from build123d import *

# Parameters (mm, degrees)
F0_R     = 34
F1_DEPTH = 5
F2_R     = 34
F2_R_2   = 3.2
F3_DEPTH = 5
F5_DEPTH = 10.001
F6_DEPTH = 4


with BuildPart() as f1:
    # F0 (on Top) → F1 (new body)
    with BuildSketch(Plane.XY):
        Circle(F0_R)
        Polygon((0, 5.34048999), (4.625, 2.670244995), (4.625, -2.670244995), (0, -5.34048999), (-4.625, -2.670244995), (-4.625, 2.670244995), align=None, mode=Mode.SUBTRACT)
    extrude(amount=F1_DEPTH)

    # F2 (on face) → F3 (join)
    with BuildSketch(Plane.XY.offset(5)):
        Circle(F2_R)
        Polygon((-4.625, -2.670244995), (-4.625, 2.670244995), (0, 5.34048999), (4.625, 2.670244995), (4.625, -2.670244995), (0, -5.34048999), align=None, mode=Mode.SUBTRACT)
        Polygon((0, 5.34048999), (-4.625, 2.670244995), (-4.625, -2.670244995), (0, -5.34048999), (4.625, -2.670244995), (4.625, 2.670244995), align=None)
        Circle(F2_R_2, mode=Mode.SUBTRACT)
    extrude(amount=F3_DEPTH)

    # F4 (on face) → F5 (cut, through all)
    with BuildSketch(Plane.XY.offset(10)):
        with BuildLine():
            ThreePointArc((34, 0), (25.9934550819, 21.9166670118), (5.7446886526, 33.5111705597))
            Line((5.7446886526, 33.5111705597), (31.8938693416, -11.7805389699))
            ThreePointArc((31.8938693416, -11.7805389699), (33.4693259389, -5.9836628575), (34, 0))
        make_face()
        with BuildLine():
            Line((-5.7446886526, -33.5111705597), (-31.8938693416, 11.7805389699))
            ThreePointArc((-31.8938693416, 11.7805389699), (-29.4448637287, -17), (-5.7446886526, -33.5111705597))
        make_face()
    extrude(amount=-F5_DEPTH, mode=Mode.SUBTRACT)

    # F4 (on face) → F6 (join)
    with BuildSketch(Plane.XY.offset(10)):
        with BuildLine():
            ThreePointArc((3.5, 33.8193731462), (1.7523288833, 33.9548132595), (0, 34))
            Line((0, 34), (0, 29.5))
            Line((0, 29.5), (3.5, 29.5))
            Line((3.5, 29.5), (3.5, 33.8193731462))
        make_face()
        with BuildLine():
            Line((-3.5, -29.5), (-3.5, -33.8193731462))
            ThreePointArc((-3.5, -33.8193731462), (-1.7523288833, -33.9548132595), (0, -34))
            Line((0, -34), (0, -29.5))
            Line((0, -29.5), (-3.5, -29.5))
        make_face()
    extrude(amount=F6_DEPTH)


solid = f1.part
Design review of the part built by this model. Coordinates are the model's own, in mm. A direction names the side the tool comes from. Coordinates: 2 decimals unless noted, no trailing zeros. Order: outer loops, then holes, each group sorted by start corner. A loop starts at its lowest first (then second) coordinate and runs counter-clockwise, first axis right, second up. Notation, with made-up numbers: M -20,13.5 L 19,13.5 A9 ccw 19,25.5 Z; hole C 68.25,36.5 d3. An arc over 180 degrees is marked long. Use a Markdown table: item, result.
(1) For P1, Ø2, axis at x = 13, y = 0, coming from the -Z side; P2, Ø2.5, axis at y = 0, z = 2, coming from the +X side; P3, Ø1, axis at x = -5.5, y = 15.5, coming from the +Z side; P4, Ø3, axis at x = 2, z = 12.5, coming from the -Y side, all flat-tipped, find the tip position at first contact; note any pin that passes through.
Worked answers:
| item | result |
|---|---|
| P1 | stops at z = 0 |
| P2 | stops at x = 25.81 |
| P3 | stops at z = 10 |
| P4 | stops at y = 29.5 |
(2) Add section A-A (z = 8.5). Give the boundary of the cut face in (x, y).
Worked answers:
| item | result |
|---|---|
| outline | M -31.89,11.78 L -5.74,-33.51 A34 ccw 31.89,-11.78 L 5.74,33.51 A34 ccw Z; hole C 0,0 d6.4 |
(3) Add section C-C (x = 7). Give the boundary of the cut face in (y, z).
Worked answers:
| item | result |
|---|---|
| outline | M -33.27,0 L 31.34,0 L 31.34,10 L -33.27,10 Z |
(4) Wall thickness on probe 1 along Y at (x, z) = (0, 6.25); probe 2 along Z at (x, y) = (-17, 5.5); probe 3 along Y at (x, z) = (3, 1.25): over which ranges is each line inside the solid? List them lowest first.
Worked answers:
| item | result |
|---|---|
| probe 1 | y = -34 to -3.2, 3.2 to 34 |
| probe 2 | z = 0 to 10 |
| probe 3 | y = -33.87 to -3.61, 3.61 to 33.87 |
(5) Add section D-D (y = 22). Give the boundary of the cut face in (x, z).
Worked answers:
| item | result |
|---|---|
| outline | M -25.92,0 L 12.39,0 L 12.39,10 L -25.92,10 Z |
(6) Draft analysis for pull direction Y (two halves, no side actions). For faces 1 (the flat face through (0, 32, 12)), 2 (the flat face through (-2, -29.5, 12)), 3 (the flat face through (-0.1, -3.5, 5)), state which applies: released by +Y, released by -Y, zero draft, split by the parting line, or undercut.
Worked answers:
| item | result |
|---|---|
| face 1 | zero draft |
| face 2 | released by +Y |
| face 3 | undercut |
(7) Add section B-B (y = 0). Give the boundary of the cut face in (x, z) (3 decimals), then the cut area to 3 significant figures.
Worked answers:
| item | result |
|---|---|
| outline | M -25.092,0 L -4.625,0 L -4.625,5 L -3.2,5 L -3.2,10 L -25.092,10 Z; M 3.2,5 L 4.625,5 L 4.625,0 L 25.092,0 L 25.092,10 L 3.2,10 Z |
| area | 424 mm2 |
(8) For faces 4 (the flat face through (2, 29.5, 12)), 5 (the flat face through (0, -32, 12)), 6 (the flat face through (-3.5, -32, 12)), 7 (the flat face through (3.5, 32, 12)), 8 (the flat face through (-2.34, 3.99, 2.46)), list the 3-axis set-ups (+Z, -Z, +X, -X, +Y, -Y) from which the entire face can be reached by the end or side of a thin tool; tool diameter is ignored.
Worked answers:
| item | result |
|---|---|
| face 4 | +Z, +X, -X, -Y |
| face 5 | +Z, +X, -Y |
| face 6 | +Z, -X, +Y, -Y |
| face 7 | +Z, +X, +Y, -Y |
| face 8 | -Z |
